Verification items for this drawing (mm, ordinates from the low corner). Round coordinates to 2 decimals unless told otherwise and drop trailing zeros. Order: outer loops, then holes, each group sorted by start corner. A loop starts at its lowest first (then second) coordinate and runs counter-clockwise, first axis right, second up. Notation, with made-up numbers: (69, 42.5) - (91, 42.5) arc R27 ccw to (91, 81.5) - close; hole circle Ø6 at (5, -14.75). An arc over 180 degrees is marked (long way). Use a Markdown table: item, result. Add a question column.
(1) Thickness scan on line 1 along Y through (x, z) = (1, 14); line 2 along Z through (x, y) = (14, 9.25); line 3 along Z through (x, y) = (10.5, 1.5). Record the ranges inside material, lowest first. Write a range as [from, to].
(2) Mould release check, pull along X, two halves, no side actions. Record for the marked faces 1, 2, 3 and 4: released by +X, released by -X, zero draft, split by the parting line, or undercut.
(3) Section check B-B on z = 12. Record the boundary of the cut face in (x, y), then the cut area to 3 significant figures.
(4) Section check D-D on y = 2.25. Record the boundary of the cut face in (x, z) (3 decimals), then the cut area to 3 significant figures.
(5) Section check A-A on x = 15. Record the boundary of the cut face in (y, z) (1 decimal), then the cut area to 3 significant figures.
(6) Section check C-C on x = 27. Record the boundary of the cut face in (y, z), then the cut area to 3 significant figures.
(7) Gauge pin test, flat ends, axial feed: P1, Ø4, axis at y = 7, z = 25.5, coming from the -X side; P2, Ø0.8, axis at x = 15.5, y = 6, coming from the +Z side; P3, Ø1, axis at y = 8.5, z = 23.5, coming from the -X side. Record the tip position at first contact, or that the pin passes through.
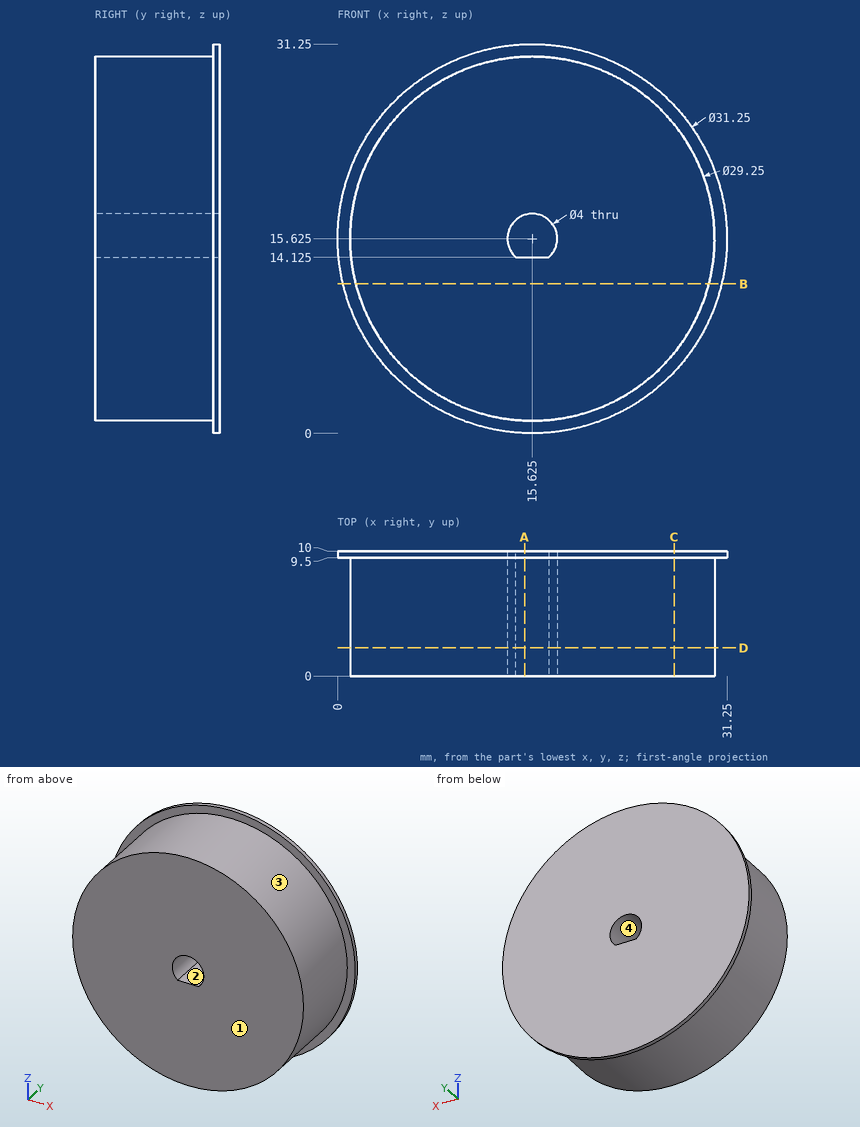
Check sheet entries:
| question | item | result |
|---|---|---|
| 1 | line 1 | y = [9.5, 10] |
| 1 | line 2 | z = [1.09, 14.46], [16.79, 30.16] |
| 1 | line 3 | z = [1.93, 29.32] |
| 2 | face 1 | zero draft |
| 2 | face 2 | undercut |
| 2 | face 3 | split by the parting line |
| 2 | face 4 | undercut |
| 3 | outline | (0.43, 9.5) - (1.46, 9.5) - (1.46, 0) - (29.79, 0) - (29.79, 9.5) - (30.82, 9.5) - (30.82, 10) - (0.43, 10) - close |
| 3 | area | 284 mm2 |
| 4 | outline | circle Ø29.25 at (15.625, 15.625); hole (14.302, 14.125) - (16.948, 14.125) arc R2 ccw (long way) to start |
| 4 | area | 660 mm2 |
| 5 | outline | (0, 1) - (9.5, 1) - (9.5, 0) - (10, 0) - (10, 14.1) - (0, 14.1) - close; (0, 17.5) - (10, 17.5) - (10, 31.2) - (9.5, 31.2) - (9.5, 30.2) - (0, 30.2) - close |
| 5 | area | 259 mm2 |
| 6 | outline | (0, 6.43) - (9.5, 6.43) - (9.5, 4.91) - (10, 4.91) - (10, 26.34) - (9.5, 26.34) - (9.5, 24.82) - (0, 24.82) - close |
| 6 | area | 185 mm2 |
| 7 | P1 | stops at x = 3.3 |
| 7 | P2 | stops at z = 30.25 |
| 7 | P3 | stops at x = 3 |
